Geometry: final body of the model. Coordinates: model frame, mm. A direction names the side the tool comes from. Coordinates: 2 decimals unless noted, no trailing zeros. Write each loop counter-clockwise with the first axis right and the second up, starting at its lowest first coordinate (ties: lowest second). Pieces come first, ordered by that corner, then holes.
from build123d import *

# Parameters (mm, degrees)
ESQUISSE1_W        = 12
ESQUISSE1_H        = 20
BOSS_EXTRU_1_DEPTH = 20
ESQUISSE2_R        = 2
BOSS_EXTRU_2_DEPTH = 4


with BuildPart() as part:
    # Esquisse1 → Boss.-Extru.1 (new body)
    with BuildSketch(Plane.XY):
        Rectangle(ESQUISSE1_W, ESQUISSE1_H)
    extrude(amount=BOSS_EXTRU_1_DEPTH)

    # Esquisse2 → Boss.-Extru.2 (add)
    with BuildSketch(Plane.XY.offset(20)):
        with BuildLine():
            Line((0, 7.5), (24.528746791, 7.5))
            ThreePointArc((24.528746791, 7.5), (31.65124579, 5), (24.528746791, 2.5))
            Line((24.528746791, 2.5), (0, 2.5))
            ThreePointArc((0, 2.5), (-2.5, 5), (0, 7.5))
        make_face()
        with Locations((27.65124579, 5)):
            Circle(ESQUISSE2_R, mode=Mode.SUBTRACT)
    extrude(amount=BOSS_EXTRU_2_DEPTH)


solid = part.part
Item 1: Set-up query: faces 1 (the flat face through (19, 5, 20)), 2 (the cylindrical face through (-2.5, 4.9, 22)), 3 (the flat face through (12, 2.5, 22)), 4 (the flat face through (12, 7.5, 22)). Return all of +Z, -Z, +X, -X, +Y, -Y with unobstructed straight access to the full face (end or side cutting, diameter ignored); none if empty.
Derived:
face 1: -Z, +X, +Y, -Y
face 2: +Z, -X
face 3: +Z, -X, -Y
face 4: +Z, -X, +Y
Item 2: Section C-C, the plane z = 18.5. Output: boundary loops of the cut face in (x, y), plus the area to 3 significant figures.
Derived:
outline: (-6, -10) - (6, -10) - (6, 10) - (-6, 10) - close
area: 240 mm2
Item 3: Section B-B, the plane x = 7.5. Output: boundary loops of the cut face in (y, z), plus the area to 3 significant figures.
Derived:
outline: (2.5, 20) - (7.5, 20) - (7.5, 24) - (2.5, 24) - close
area: 20.0 mm2
Item 4: Pin query (flat end, axial travel): pin 1 (4.5 mm diameter, centred on x = 13, z = 22, fed in from -Y); pin 2 (4.5 mm diameter, centred on x = 27.65, y = 5, fed in from -Z); pin 3 (6 mm diameter, centred on x = -1, y = -0.5, fed in from +Z). Return the tip coordinate at first contact, or that it passes through.
Derived:
pin 1: stops at y = 2.5
pin 2: stops at z = 20
pin 3: stops at z = 20
Item 5: Section A-A, the plane y = 5. Output: boundary loops of the cut face in (x, z), plus the area to 3 significant figures.
Derived:
outline: (-6, 0) - (6, 0) - (6, 20) - (25.65, 20) - (25.65, 24) - (-2.5, 24) - (-2.5, 20) - (-6, 20) - close; (29.65, 20) - (31.65, 20) - (31.65, 24) - (29.65, 24) - close
area: 361 mm2
Item 6: Pull-direction query (Y, two-part tool) for faces 5 (the flat face through (0, 10, 10)), 6 (the flat face through (6, 0, 10)), 7 (the cylindrical face through (25.653, 5.088, 21.972)); classes: released by +Y, released by -Y, zero draft, split by the parting line, or undercut.
Derived:
face 5: released by +Y
face 6: zero draft
face 7: undercut
Item 7: Material intervals for probe 1 along Z at (x, y) = (1, -7); probe 2 along X at (y, z) = (-6.75, 10.75); probe 3 along Z at (x, y) = (9, 3), sorted ascending.
Derived:
probe 1: z = 0 to 20
probe 2: x = -6 to 6
probe 3: z = 20 to 24
